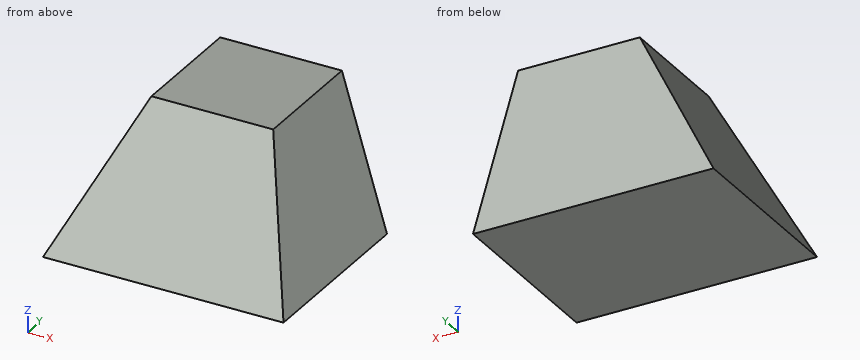
from build123d import *

# Parameters (mm, degrees)
F0_W     = 800
F0_H     = 610
F1_DEPTH = 250
F3_DEPTH = 610.001
F6_DEPTH = 800.001


with BuildPart() as f1:
    # F0 (on Top) → F1 (new body, symmetric)
    with BuildSketch(Plane.XY):
        Rectangle(F0_W, F0_H)
    extrude(amount=F1_DEPTH, both=True)

    # F2 (on face) → F3 (cut, through all)
    with BuildSketch(Plane.XZ.offset(305)):
        Polygon((-155, 250), (-400, 250), (-400, -250), align=None)
        Polygon((400, 250), (250, 250), (400, -250), align=None)
    extrude(amount=-F3_DEPTH, mode=Mode.SUBTRACT)

    # F5 (on offset) → F6 (cut, through all)
    with BuildSketch(Plane.YZ.offset(-400)):
        Polygon((-305, -250), (-100, 250), (-305, 250), align=None)
    extrude(amount=F6_DEPTH, mode=Mode.SUBTRACT)


solid = f1.part
Verification items for the finished model (mm, model axes). Give positions to 0.01 mm unless a question says otherwise; leave off trailing zeros. Loops run counter-clockwise (first coordinate to the right, second up) from the corner with the lowest first, then second, coordinate; pieces in that order, holes last.
1) Sectioned sample at B-B, the plane y = -85. Enter the section's corners in (x, z).
2) Depth check by flat-ended pin: pin 1 Ø2 at (x, z) = (-303.5, -65) entering from -Y; pin 2 Ø5 at (x, z) = (-32.5, -32) entering from -Y (3 decimals); pin 3 Ø6 at (y, z) = (114, 95) entering from -X. Enter the tip coordinate at first touch or a pass-through.
3) Thickness scan on line 1 along X through (y, z) = (197.5, -108.5) (3 decimals); line 2 along Y through (x, z) = (-18, 125); line 3 along Z through (x, y) = (272, -229). Record the ranges inside material, lowest first.
4) Sectioned sample at A-A, the plane z = 14. Enter the section's corners in (x, y).
Answers:
1. outline: (-400, -250) - (400, -250) - (250, 250) - (-155, 250) - close
2. pin 1: stops at y = -229.56
2. pin 2: stops at y = -216.645
2. pin 3: stops at x = -232.42
3. line 1: x = -330.665 to 357.55
3. line 2: y = -151.25 to 305
3. line 3: z = -250 to -64.63
4. outline: (-270.64, -196.76) - (320.8, -196.76) - (320.8, 305) - (-270.64, 305) - close
